Geometry check sheet. Reference: the model listing, model coordinates, mm. A direction names the side the tool comes from. Coordinates: 2 decimals unless noted, no trailing zeros. Order: outer loops, then holes, each group sorted by start corner. A loop starts at its lowest first (then second) coordinate and runs counter-clockwise, first axis right, second up. Notation, with made-up numbers: (-26, 84) -> (25, 84) arc R29 cw to (25, 107) -> close; hole circle Ø9 at (51.25, 29.25). An arc over 180 degrees is marked (long way). Answer in a Markdown table with one row per item. Add a question column.
```python
from build123d import *

# Parameters (mm, degrees)
F0_W     = 58
F0_H     = 61
F0_R     = 1.5
F0_W_2   = 38
F0_H_2   = 25
F0_W_3   = 3
F0_H_3   = 7
F0_R_2   = 2.5
F1_DEPTH = 5
F2_W     = 40
F2_H     = 27
F2_W_2   = 38
F2_H_2   = 25
F3_DEPTH = 2


with BuildPart() as f1:
    # F0 (on Top) → F1 (new body)
    with BuildSketch(Plane.XY):
        with Locations((29, -30.5)):
            Rectangle(F0_W, F0_H)
        with Locations((3.5, -57.5)):
            Circle(F0_R, mode=Mode.SUBTRACT)
        with Locations((20.599063, -52.302592)):
            Circle(F0_R, mode=Mode.SUBTRACT)
        with Locations((13.542605, -44.172324)):
            Circle(F0_R, mode=Mode.SUBTRACT)
        with Locations((40.279038, -44.172324)):
            Circle(F0_R, mode=Mode.SUBTRACT)
        with Locations((26, -18.5)):
            Rectangle(F0_W_2, F0_H_2, mode=Mode.SUBTRACT)
        with Locations((49.58617, -27.5)):
            Rectangle(F0_W_3, F0_H_3, mode=Mode.SUBTRACT)
        with Locations((49.604766, -18.574871)):
            Circle(F0_R_2, mode=Mode.SUBTRACT)
        with Locations((54.5, -3.5)):
            Circle(F0_R, mode=Mode.SUBTRACT)
    extrude(amount=F1_DEPTH)

    # F2 (on face) → F3 (join)
    with BuildSketch(Plane.XY.offset(5)):
        with Locations((26, -18.5)):
            Rectangle(F2_W, F2_H)
        with Locations((26, -18.5)):
            Rectangle(F2_W_2, F2_H_2, mode=Mode.SUBTRACT)
    extrude(amount=F3_DEPTH)


solid = f1.part
```
(1) Mould release check, pull along Y, two halves, no side actions. Record for faces 1 (the face through (26, -6, 3)), 2 (the face through (58, -31, 2)), 3 (the face through (29, -61, 2)), 4 (the face through (45, -19, 3)): +Y half, -Y half, draft (parallel to the pull), parting line (faces both ways), or undercut.
(2) Cross-section at B-B (x = 54.5). Enter the section's corners in (y, z), plus the area to 3 significant figures.
(3) Cross-section at A-A (y = -28.5). Enter the section's corners in (x, z).
(4) Scan lines: line 1 along Y through (x, z) = (18, 4.75); line 2 along Y through (x, z) = (38, 6); line 3 along X through (y, z) = (-13, 1.25). Record each from-to range of solid material in increasing order.
(5) Cross-section at C-C (y = -3.5). Enter the section's corners in (x, z), plus the area to 3 significant figures.
(6) Access from +Z, -Z, +X, -X, +Y, -Y to the whole of each face (thin tool, end or side, straight path). Record for faces 5 (the face through (50, -24, 2)), 6 (the face through (6, -19, 6)), 7 (the face through (26, -5, 6)).
(7) Go/stop test with flat-tipped pins: P1, Ø5, axis at x = 20.6, y = -52.3, coming from the +Z side; P2, Ø1, axis at y = -24, z = 6.5, coming from the -X side; P3, Ø0.6, axis at x = 19.5, z = 6, coming from the -Y side. Record where each tip stops, or that it passes through.
(8) Cross-section at D-D (z = 1.5). Give the number of separate pieces and of enclosed holes in the cut face, plus the area to 3 significant figures.
Checks:
| question | item | result |
|---|---|---|
| 1 | face 1 | undercut |
| 1 | face 2 | draft |
| 1 | face 3 | -Y half |
| 1 | face 4 | undercut |
| 2 | outline | (-61, 0) -> (-5, 0) -> (-5, 5) -> (-61, 5) -> close; (-2, 0) -> (0, 0) -> (0, 5) -> (-2, 5) -> close |
| 2 | area | 290 mm² |
| 3 | outline | (0, 0) -> (7, 0) -> (7, 7) -> (6, 7) -> (6, 5) -> (0, 5) -> close; (45, 0) -> (48.09, 0) -> (48.09, 5) -> (46, 5) -> (46, 7) -> (45, 7) -> close; (51.09, 0) -> (58, 0) -> (58, 5) -> (51.09, 5) -> close |
| 4 | line 1 | -61 to -31, -6 to 0 |
| 4 | line 2 | -32 to -31, -6 to -5 |
| 4 | line 3 | 0 to 7, 45 to 58 |
| 5 | outline | (0, 0) -> (53, 0) -> (53, 5) -> (0, 5) -> close; (56, 0) -> (58, 0) -> (58, 5) -> (56, 5) -> close |
| 5 | area | 275 mm² |
| 6 | face 5 | +Z, -Z |
| 6 | face 6 | +Z, -X, +Y, -Y |
| 6 | face 7 | +Z, +X, -X, +Y |
| 7 | P1 | z = 5 |
| 7 | P2 | x = 6 |
| 7 | P3 | y = -32 |
| 8 | separate pieces | 1 |
| 8 | enclosed holes | 8 |
| 8 | area | 2,510 mm² |
